from build123d import *

# Parameters (mm, degrees)
F1_DEPTH = 19.05
F2_R     = 25.4
F3_DEPTH = 9.525
F4_R     = 12.7


with BuildPart() as f1:
    # F0 (on Top) → F1 (new body)
    with BuildSketch(Plane.XY):
        Polygon((-228.6, -44.45), (101.6, -44.45), (101.6, -19.05), (228.6, -19.05), (228.6, 19.05), (101.6, 19.05), (101.6, 44.45), (-228.6, 44.45), align=None)
    extrude(amount=F1_DEPTH)

    # F2 (on face) → F3 (cut)
    with BuildSketch(Plane.XY.offset(19.05)):
        with Locations((-177.8, 0)):
            Circle(F2_R)
        with Locations((-101.6, 0)):
            Circle(F2_R)
        with Locations((-25.4, 0)):
            Circle(F2_R)
        with Locations((50.8, 0)):
            Circle(F2_R)
    extrude(amount=-F3_DEPTH, mode=Mode.SUBTRACT)

    # F4
    f4_edges = [f1.edges().sort_by_distance(p)[0] for p in [
        (-228.6, -44.45, 9.525),
        (101.6, -44.45, 9.525),
        (101.6, 44.45, 9.525),
        (228.6, -19.05, 9.525),
        (228.6, 19.05, 9.525),
        (-228.6, 44.45, 9.525),
    ]]
    fillet(f4_edges, radius=F4_R)


solid = f1.part
Can you work these out from the model? Positions are in its coordinate system, mm. A direction names the side the tool comes from. Give positions to 0.01 mm unless a question says otherwise; leave off trailing zeros. Order: outer loops, then holes, each group sorted by start corner. A loop starts at its lowest first (then second) coordinate and runs counter-clockwise, first axis right, second up. Notation, with made-up numbers: M -11.5,21 L 29.5,21 A27 ccw 29.5,41 Z; hole C 80,14 d10. An arc over 180 degrees is marked long. Use one line per item in the form item = value.
Item 1: Thinking about a two-plate mould opening in Y: for faces 1 (the cylindrical face through (224.98, 15.23, 9.66)), 2 (the cylindrical face through (-1.173, 7.629, 14.354)), 3 (the flat face through (-26, 0, 9.525)), 4 (the flat face through (158, -19.05, 9)), which applies, pulls with the +Y half, pulls with the -Y half, needs draft (parallel to the pull), parting line crosses it, or undercut?
Values follow:
face_1 = pulls with the +Y half
face_2 = undercut
face_3 = undercut
face_4 = pulls with the -Y half
Item 2: If I drill on line 1 along X through (y, z) = (-16, 16); line 2 along Y through (x, z) = (-25.4, 16); line 3 along Z through (x, y) = (-25.5, -14) (3 decimals), over which ranges is the centre line in solid material (lowest first)? Write a range as [from, to].
Values follow:
line_1 = [-228.6, -197.53], [-158.07, -121.33], [-81.87, -45.13], [-5.67, 31.07], [70.53, 224.16]
line_2 = [-44.45, -25.4], [25.4, 44.45]
line_3 = [0, 9.525]
Item 3: If we section it at A-A, the plane z = 14.75: Write out the boundary of the cut face in (x, y), and give its area (3 significant figures).
Values follow:
outline = M -228.6,-31.75 A12.7 ccw -215.9,-44.45 L 88.9,-44.45 A12.7 ccw 101.6,-31.75 L 101.6,-19.05 L 215.9,-19.05 A12.7 ccw 228.6,-6.35 L 228.6,6.35 A12.7 ccw 215.9,19.05 L 101.6,19.05 L 101.6,31.75 A12.7 ccw 88.9,44.45 L -215.9,44.45 A12.7 ccw -228.6,31.75 Z; hole C -177.8,0 d50.8; hole C -101.6,0 d50.8; hole C -25.4,0 d50.8; hole C 50.8,0 d50.8
area = 25,900 mm^2
Item 4: If we section it at B-B, the plane x = 50.8: Write out the boundary of the cut face in (y, z) (3 decimals), and give its area (3 significant figures).
Values follow:
outline = M -44.45,0 L 44.45,0 L 44.45,19.05 L 25.4,19.05 L 25.4,9.525 L -25.4,9.525 L -25.4,19.05 L -44.45,19.05 Z
area = 1,210 mm^2
Item 5: If we section it at C-C, the plane y = 13.5: Write out the boundary of the cut face in (x, z) (3 decimals).
Values follow:
outline = M -228.6,0 L 226.396,0 L 226.396,19.05 L 72.315,19.05 L 72.315,9.525 L 29.285,9.525 L 29.285,19.05 L -3.885,19.05 L -3.885,9.525 L -46.915,9.525 L -46.915,19.05 L -80.085,19.05 L -80.085,9.525 L -123.115,9.525 L -123.115,19.05 L -156.285,19.05 L -156.285,9.525 L -199.315,9.525 L -199.315,19.05 L -228.6,19.05 Z
Item 6: Will these pins go through, and if not, where does the flat tip stop? pin 1 Ø9.5 at (x, z) = (172.5, 14) entering from +Y; pin 2 Ø3 at (x, z) = (142.5, 7) entering from -Y; pin 3 Ø10 at (y, z) = (-26.5, 7) entering from +X.
Values follow:
pin_1 = 19.05
pin_2 = -19.05
pin_3 = 101.6
Item 7: If we section it at D-D, the plane x = -14: Write out the boundary of the cut face in (y, z) (3 decimals), and give its area (3 significant figures).
Values follow:
outline = M -44.45,0 L 44.45,0 L 44.45,19.05 L 22.698,19.05 L 22.698,9.525 L -22.698,9.525 L -22.698,19.05 L -44.45,19.05 Z
area = 1,260 mm^2
Item 8: For faces 5 (the flat face through (101.6, -25, 9)), 6 (the flat face through (101.6, 25, 9)), 7 (the cylindrical face through (-77.373, 7.629, 14.354)), which set-ups out of +Z, -Z, +X, -X, +Y, -Y let a thin tool reach every point of the face, with its end or its side?
Values follow:
face_5 = +Z, -Z, +X, -Y
face_6 = +Z, -Z, +X, +Y
face_7 = +Z
